from build123d import *

# Parameters (mm, degrees)
SKETCH1_W           = 19.05
SKETCH1_H           = 25.4
BOSS_EXTRUDE1_DEPTH = 6.35
SKETCH2_W           = 9.525
SKETCH2_H           = 25.4
CUT_EXTRUDE1_DEPTH  = 3.175
CUT_EXTRUDE2_DEPTH  = 26.4
CUT_EXTRUDE3_DEPTH  = 4.175
FILLET1_R           = 0.254
CHAMFER1_SIZE       = 0.254


with BuildPart() as part:
    # Sketch1 → Boss-Extrude1 (new body)
    with BuildSketch(Plane(origin=(0, 0, 0), x_dir=(1, 0, 0), z_dir=(0, 1, 0))):
        with Locations((9.525, 12.7)):
            Rectangle(SKETCH1_W, SKETCH1_H)
    extrude(amount=BOSS_EXTRUDE1_DEPTH)

    # Sketch2 → Cut-Extrude1 (cut)
    with BuildSketch(Plane(origin=(0, 6.35, 0), x_dir=(1, 0, 0), z_dir=(0, 1, 0))):
        with Locations((4.7625, 12.7)):
            Rectangle(SKETCH2_W, SKETCH2_H)
    extrude(amount=-CUT_EXTRUDE1_DEPTH, mode=Mode.SUBTRACT)

    # Sketch3 → Cut-Extrude2 (cut, through all)
    with BuildSketch(Plane.XY):
        Polygon((8.608456448, 0), (9.525, 1.5875), (10.441543552, 0), align=None)
    extrude(amount=-CUT_EXTRUDE2_DEPTH, mode=Mode.SUBTRACT)

    # Sketch4 → Cut-Extrude3 (cut, through all)
    with BuildSketch(Plane(origin=(0, 3.175, 0), x_dir=(1, 0, 0), z_dir=(0, 1, 0))):
        with BuildLine():
            Line((6.35, 22.225), (6.35, 17.145))
            ThreePointArc((6.35, 17.145), (4.7625, 15.5575), (3.175, 17.145))
            Line((3.175, 17.145), (3.175, 22.225))
            ThreePointArc((3.175, 22.225), (4.7625, 23.8125), (6.35, 22.225))
        make_face()
        with BuildLine():
            Line((6.35, 8.255), (6.35, 3.175))
            ThreePointArc((6.35, 3.175), (4.7625, 1.5875), (3.175, 3.175))
            Line((3.175, 3.175), (3.175, 8.255))
            ThreePointArc((3.175, 8.255), (4.7625, 9.8425), (6.35, 8.255))
        make_face()
    extrude(amount=-CUT_EXTRUDE3_DEPTH, mode=Mode.SUBTRACT)

    # Fillet1
    fillet1_edges = [part.edges().sort_by_distance(p)[0] for p in [
        (19.05, 6.35, -12.7),
        (14.2875, 6.35, -25.4),
        (14.2875, 6.35, 0),
        (0, 1.5875, -25.4),
        (0, 1.5875, 0),
        (0, 3.175, -12.7),
        (4.7625, 3.175, -25.4),
        (9.525, 3.175, -12.7),
        (9.525, 4.7625, -25.4),
        (4.7625, 3.175, 0),
        (9.525, 4.7625, 0),
        (9.525, 6.35, -12.7),
        (4.304228224, 0, -25.4),
        (14.745771776, 0, 0),
        (10.441543552, 0, -12.7),
        (9.066728224, 0.79375, -25.4),
        (8.608456448, 0, -12.7),
        (9.983271776, 0.79375, -25.4),
        (9.983271776, 0.79375, 0),
        (9.066728224, 0.79375, 0),
        (14.745771776, 0, -25.4),
        (19.05, 0, -12.7),
        (4.304228224, 0, 0),
        (0, 0, -12.7),
        (19.05, 3.175, -25.4),
        (19.05, 3.175, 0),
    ]]
    fillet(fillet1_edges, radius=FILLET1_R)

    # Chamfer1
    chamfer1_edges = [part.edges().sort_by_distance(p)[0] for p in [
        (4.7625, 0, -23.8125),
        (6.35, 0, -19.685),
        (4.7625, 0, -15.5575),
        (3.175, 0, -19.685),
        (4.7625, 3.175, -23.8125),
        (3.175, 3.175, -19.685),
        (4.7625, 3.175, -15.5575),
        (6.35, 3.175, -19.685),
        (4.7625, 0, -9.8425),
        (6.35, 0, -5.715),
        (4.7625, 0, -1.5875),
        (3.175, 0, -5.715),
        (4.7625, 3.175, -9.8425),
        (3.175, 3.175, -5.715),
        (4.7625, 3.175, -1.5875),
        (6.35, 3.175, -5.715),
    ]]
    chamfer(chamfer1_edges, length=CHAMFER1_SIZE)


solid = part.part
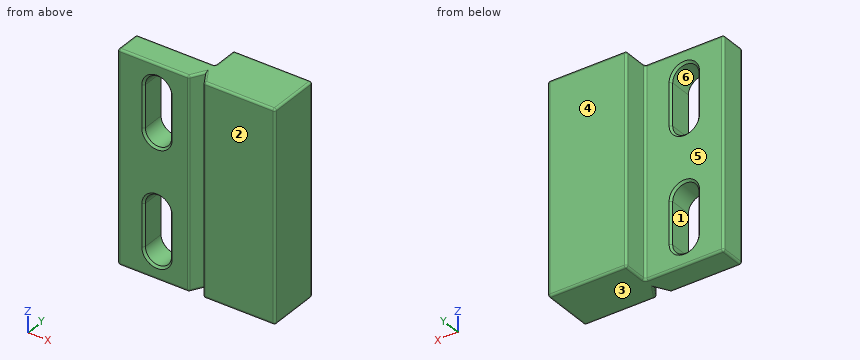
The listing builds one solid part. Answer for the finished solid, in the listing's coordinates (mm). Face numbers are marked on the shaded views. A direction names the side the tool comes from. Coordinates: 2 decimals unless noted, no trailing zeros. Write each loop counter-clockwise with the first axis right and the second up, starting at its lowest first coordinate (ties: lowest second). Pieces come first, ordered by that corner, then holes. Notation, with made-up numbers: (-17.75, -8.75) - (2.25, -8.75) arc R18 cw to (2.25, 5.25) - close; hole circle Ø1 at (56, 80). An arc over 180 degrees is marked (long way). Return JSON: item names as keys, results as strings.
1. For a pull along Z with two mould halves and no side action, classify the marked faces 1, 2 and 3 as +Z half, -Z half, draft (parallel to the pull), parting line (faces both ways), or undercut.
Final values:
{"face 1": "undercut", "face 2": "draft", "face 3": "-Z half"}
2. This flat-tipped pin is pushed along its axis until it touches: pin 1 Ø3 at (y, z) = (4.5, -9.5) entering from -X. Where does it stop, or does it pass through?
Final values:
{"pin 1": "x = 0.01"}
3. The part is cut by section B-B on x = 2.25. Determine the outline of the cut face in (y, z) (3 decimals), then the cut area to 3 significant figures.
Final values:
{"outline": "(0, -25.146) arc R0.254 ccw to (0.254, -25.4) - (2.921, -25.4) arc R0.254 ccw to (3.175, -25.146) - (3.175, -0.254) arc R0.254 ccw to (2.921, 0) - (0.254, 0) arc R0.254 ccw to (0, -0.254) - close", "area": "80.6 mm^2"}
4. Consider line 1 along X through (y, z) = (1.75, -19.75) (3 decimals); line 2 along X through (y, z) = (1.25, -16.5); line 3 along X through (y, z) = (5.25, -15) (3 decimals). Determine where each line is inside the solid, lowest interval first.
Final values:
{"line 1": "0 to 3.175, 6.35 to 19.05", "line 2": "0 to 3.31, 6.21 to 9.33, 9.72 to 19.05", "line 3": "9.525 to 19.05"}
5. The part is cut by section C-C on y = 5. Determine the outline of the cut face in (x, z) (3 decimals), then the cut area to 3 significant figures.
Final values:
{"outline": "(9.525, -25.146) arc R0.254 ccw to (9.779, -25.4) - (18.796, -25.4) arc R0.254 ccw to (19.05, -25.146) - (19.05, -0.254) arc R0.254 ccw to (18.796, 0) - (9.779, 0) arc R0.254 ccw to (9.525, -0.254) - close", "area": "242 mm^2"}
6. Which of the six approach directions +Z, -Z, +X, -X, +Y, -Y give full straight-line access (tool end or side, diameter ignored) to the marked faces 4, 5 and 6?
Final values:
{"face 4": "+Z, -Z, +X, -X, +Y", "face 5": "+Z, -Z, -X, +Y", "face 6": "+Y, -Y"}
